Here's the drawing with two shaded views (mm, measured from the low corner). I have some questions. Coordinates: 2 decimals unless noted, no trailing zeros. Order: outer loops, then holes, each group sorted by start corner. A loop starts at its lowest first (then second) coordinate and runs counter-clockwise, first axis right, second up. Notation, with made-up numbers: (-11, 62) -> (6, 62) arc R36 cw to (6, 101) -> close; hole circle Ø6 at (-20, 49.5). An arc over 180 degrees is marked (long way). Answer as a JSON object with one key per item and string values. Group by question number.
(1) I want a section at A-A, the plane z = 11. List the corners of the cut face in (x, y) for me, plus the area to 3 significant figures.
(2) I need wall thicknesses on line 1 (X direction, y = 9.25, z = 37.5); line 2 (Z direction, x = 115, y = 3.5); line 3 (X direction, y = 8.5, z = 26.5). Which ranges of each line are inside material? Lowest first, please.
(3) I want a section at D-D, the plane y = 6.5. List the corners of the cut face in (x, z) for me.
(4) I want a section at C-C, the plane x = 8.5. List the corners of the cut face in (y, z) for me.
(5) If we mould it in two halves opening along X, with no side actions, what happens to the marked faces 1, 2 and 3? For each: pulls with the +X half, pulls with the -X half, needs draft (parallel to the pull), parting line crosses it, or undercut.
(6) I want a section at B-B, the plane y = 14.25. List the corners of the cut face in (x, z) for me.
(7) For pin 1 (0.9 mm diameter, centred on x = 65, z = 20, fed in from -Y), with a flat end and sliding along its axis, tell me the tip position at first contact or that it passes through.
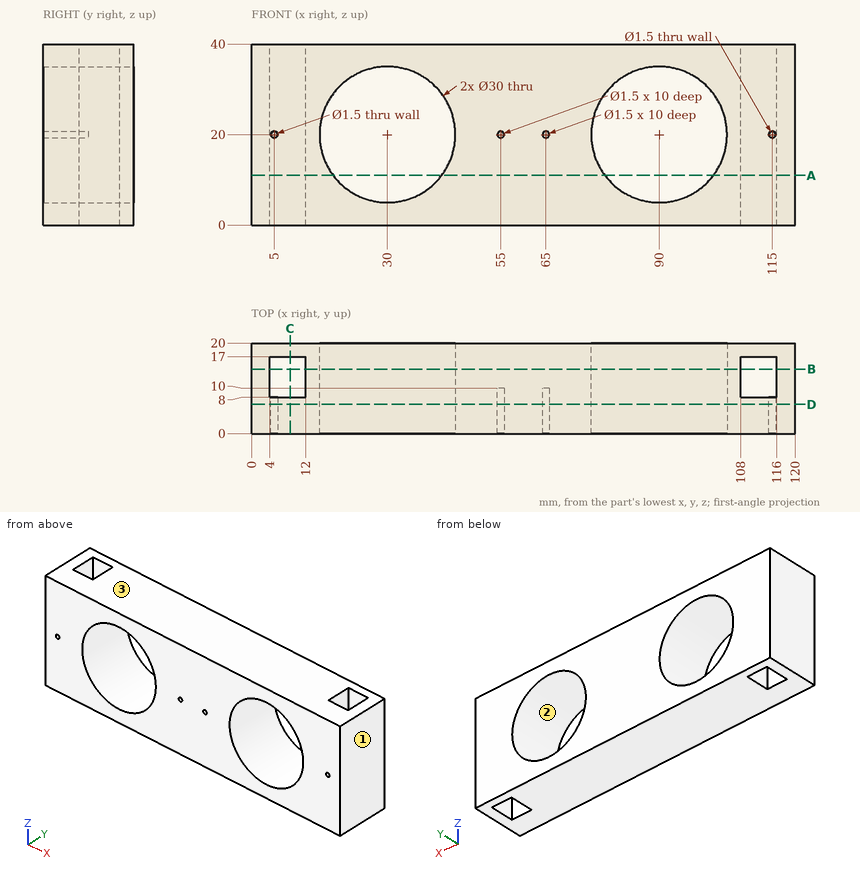
Computed values:
{
 "1": {"outline": "(0, 0) -> (18, 0) -> (18, 20) -> (0, 20) -> close; (42, 0) -> (78, 0) -> (78, 20) -> (42, 20) -> close; (102, 0) -> (120, 0) -> (120, 20) -> (102, 20) -> close; hole (4, 8) -> (12, 8) -> (12, 17) -> (4, 17) -> close; hole (108, 8) -> (116, 8) -> (116, 17) -> (108, 17) -> close", "area": "1,300 mm2"},
 "2": {"line 1": "x = 0 to 4, 12 to 108, 116 to 120", "line 2": "z = 0 to 19.25, 20.75 to 40", "line 3": "x = 0 to 4, 12 to 16.48, 43.52 to 76.48, 103.52 to 108, 116 to 120"},
 "3": {"outline": "(0, 0) -> (120, 0) -> (120, 40) -> (0, 40) -> close; hole circle Ø1.5 at (5, 20); hole circle Ø30 at (30, 20); hole circle Ø1.5 at (55, 20); hole circle Ø1.5 at (65, 20); hole circle Ø30 at (90, 20); hole circle Ø1.5 at (115, 20)"},
 "4": {"outline": "(0, 0) -> (8, 0) -> (8, 40) -> (0, 40) -> close; (17, 0) -> (20, 0) -> (20, 40) -> (17, 40) -> close"},
 "5": {"face 1": "pulls with the +X half", "face 2": "undercut", "face 3": "needs draft"},
 "6": {"outline": "(0, 0) -> (4, 0) -> (4, 40) -> (0, 40) -> close; (12, 0) -> (108, 0) -> (108, 40) -> (12, 40) -> close; (116, 0) -> (120, 0) -> (120, 40) -> (116, 40) -> close; hole circle Ø30 at (30, 20); hole circle Ø30 at (90, 20)"},
 "7": {"pin 1": "stops at y = 10"}
}
